The listing builds one solid part. Answer for the finished solid, in the listing's coordinates (mm). Round coordinates to 2 decimals unless told otherwise and drop trailing zeros. Write each loop counter-clockwise with the first axis right and the second up, starting at its lowest first coordinate (ties: lowest second). Pieces come first, ordered by that corner, then holes.
(1) A cutting plane is placed at B-B, the plane x = -24.5. Give the vertices of the cut face in (y, z).
(2) This flat-tipped pin is pushed along its axis until it touches: pin 1 Ø4 at (x, z) = (63.74, -44.39) entering from +Y. Where does it stop, or does it pass through?
(3) The mould has two halves that part along Z. Classify faces 1 (the face through (39.971, 0.394, -76.843)), 2 (the face through (65.297, 0.394, -75.89)), 3 (the face through (-58.667, 0.394, -87.399)), 4 (the face through (-58.511, 0.394, -19.757)): +Z half, -Z half, draft (parallel to the pull), parting line (faces both ways), or undercut.
(4) Find the intervals of material crossed by probe 1 along X at (y, z) = (0.4, -76); probe 2 along X at (y, z) = (0.25, -30); probe 3 along X at (y, z) = (0.25, 9), in increasing order.
(5) A cutting plane is placed at A-A, the plane y = 0.5. Give the number of separate pieces and of enclosed holes in the cut face, and give its area (3 significant figures).
(6) A cutting plane is placed at C-C, the plane z = 38. Give the vertices of the cut face in (x, y).
from build123d import *

# Parameters (mm, degrees)
SKETCH_1_R      = 1.57
SKETCH_1_R_2    = 2
SKETCH_1_R_3    = 2.5
EXTRUDE_1_DEPTH = 0.8


with BuildPart() as part:
    # 草图1 → 凸台-拉伸1 (new body)
    with BuildSketch(Plane(origin=(0, 0, 0), x_dir=(1, 0, 0), z_dir=(0, 1, 0))):
        with BuildLine():
            Line((-51.518366865, 90.405716602), (66.740135943, 90.405716602))
            ThreePointArc((66.740135943, 90.405716602), (73.811203755, 87.476784413), (76.740135943, 80.405716602))
            Line((76.740135943, 80.405716602), (76.740135943, 30.195483944))
            Line((76.740135943, 30.195483944), (76.740135943, -39.991264165))
            ThreePointArc((76.740135943, -39.991264165), (73.811203755, -47.062331977), (66.740135943, -49.991264165))
            Line((66.740135943, -49.991264165), (35.120135943, -49.991264165))
            Line((35.120135943, -49.991264165), (8.739202574, -49.991264165))
            ThreePointArc((8.739202574, -49.991264165), (1.668134763, -47.062331977), (-1.260797426, -39.991264165))
            Line((-1.260797426, -39.991264165), (-1.260797426, 6.905716602))
            ThreePointArc((-1.260797426, 6.905716602), (-4.189729614, 13.976784413), (-11.260797426, 16.905716602))
            Line((-11.260797426, 16.905716602), (-51.518366865, 16.905716602))
            ThreePointArc((-51.518366865, 16.905716602), (-58.589434677, 19.83464879), (-61.518366865, 26.905716602))
            Line((-61.518366865, 26.905716602), (-61.518366865, 80.405716602))
            ThreePointArc((-61.518366865, 80.405716602), (-58.589434677, 87.476784413), (-51.518366865, 90.405716602))
        make_face()
        with Locations(Location((-36.068366865, 77.755716602, 0), (0, 0, 270))):
            Circle(SKETCH_1_R, mode=Mode.SUBTRACT)
        with Locations(Location((23.290135943, 75.685716602, 0), (0, 0, 270))):
            Circle(SKETCH_1_R, mode=Mode.SUBTRACT)
        with Locations(Location((38.910135943, 75.685716602, 0), (0, 0, 270))):
            Circle(SKETCH_1_R, mode=Mode.SUBTRACT)
        with Locations(Location((48.120135943, 75.685716602, 0), (0, 0, 270))):
            Circle(SKETCH_1_R, mode=Mode.SUBTRACT)
        with Locations(Location((63.740135943, 75.685716602, 0), (0, 0, 270))):
            Circle(SKETCH_1_R, mode=Mode.SUBTRACT)
        with Locations(Location((-37.618366865, 29.855716602, 0), (0, 0, 270))):
            Circle(SKETCH_1_R, mode=Mode.SUBTRACT)
        with Locations(Location((14.081633135, 34.955716602, 0), (0, 0, 270))):
            Circle(SKETCH_1_R, mode=Mode.SUBTRACT)
        with Locations(Location((14.081633135, 61.755716602, 0), (0, 0, 270))):
            Circle(SKETCH_1_R, mode=Mode.SUBTRACT)
        with Locations(Location((23.290135943, 44.385716602, 0), (0, 0, 270))):
            Circle(SKETCH_1_R, mode=Mode.SUBTRACT)
        with Locations(Location((38.910135943, 44.385716602, 0), (0, 0, 270))):
            Circle(SKETCH_1_R, mode=Mode.SUBTRACT)
        with Locations(Location((48.120135943, 44.385716602, 0), (0, 0, 270))):
            Circle(SKETCH_1_R, mode=Mode.SUBTRACT)
        with Locations(Location((63.740135943, 44.385716602, 0), (0, 0, 270))):
            Circle(SKETCH_1_R, mode=Mode.SUBTRACT)
        with Locations(Location((13.239202574, -9.491264165, 0), (0, 0, 270))):
            Circle(SKETCH_1_R_2, mode=Mode.SUBTRACT)
        with Locations(Location((62.239202574, -9.491264165, 0), (0, 0, 270))):
            Circle(SKETCH_1_R_2, mode=Mode.SUBTRACT)
        with Locations(Location((-55.518366865, 84.405716602, 0), (0, 0, 270))):
            Circle(SKETCH_1_R_3, mode=Mode.SUBTRACT)
        with Locations(Location((70.740135943, 84.405716602, 0), (0, 0, 270))):
            Circle(SKETCH_1_R_3, mode=Mode.SUBTRACT)
        with Locations(Location((70.740135943, -43.991264165, 0), (0, 0, 270))):
            Circle(SKETCH_1_R_3, mode=Mode.SUBTRACT)
    extrude(amount=EXTRUDE_1_DEPTH)


solid = part.part
Solutions:
1. outline: (0, -90.41) - (0.8, -90.41) - (0.8, -16.91) - (0, -16.91) - close
2. pin 1: stops at y = 0.8
3. face 1: undercut
3. face 2: undercut
3. face 3: -Z half
3. face 4: +Z half
4. probe 1: x = -61.52 to 21.75, 24.83 to 37.37, 40.45 to 46.58, 49.66 to 62.2, 65.28 to 76.74
4. probe 2: x = -61.52 to -39.18, -36.06 to 76.74
4. probe 3: x = -1.26 to 11.3, 15.18 to 60.3, 64.18 to 76.74
5. separate pieces: 1
5. enclosed holes: 17
5. area: 15,100 mm2
6. outline: (-1.26, 0) - (76.74, 0) - (76.74, 0.8) - (-1.26, 0.8) - close
